```python
from build123d import *

# Parameters (mm, degrees)
SKETCH1_W           = 3.175
SKETCH1_H           = 50.8
BOSS_EXTRUDE1_DEPTH = 38.1
SKETCH3_R           = 3.175
CUT_EXTRUDE1_DEPTH  = 38.1
FILLET1_R           = 12.7


with BuildPart() as part:
    # Sketch1 → Boss-Extrude1 (new body)
    with BuildSketch(Plane.XY):
        with Locations((17.4625, -24.384)):
            Rectangle(SKETCH1_W, SKETCH1_H)
    extrude(amount=BOSS_EXTRUDE1_DEPTH)

    # Sketch3 → Cut-Extrude1 (cut)
    with BuildSketch(Plane.ZY.offset(-15.875)):
        with Locations((19.05, -24.384)):
            Circle(SKETCH3_R)
    extrude(amount=-CUT_EXTRUDE1_DEPTH, mode=Mode.SUBTRACT)

    # Fillet1
    fillet1_edges = [part.edges().sort_by_distance(p)[0] for p in [
        (17.4625, -49.784, 38.1),
        (17.4625, 1.016, 38.1),
    ]]
    fillet(fillet1_edges, radius=FILLET1_R)


solid = part.part
```
Source: CAD feature listing. Evaluate the final solid. Frame: model axes, mm. Round coordinates to 2 decimals unless told otherwise and drop trailing zeros. Write each loop counter-clockwise with the first axis right and the second up, starting at its lowest first coordinate (ties: lowest second). Pieces come first, ordered by that corner, then holes. Notation, with made-up numbers: M 50,-12.75 L 100,-12.75 A29 ccw 100,10.25 Z; hole C 4,-7 d4. An arc over 180 degrees is marked long. Answer as a JSON object with one key per item and string values. Group by question number.
(1) First-contact query: pin 1 (10 mm diameter, centred on y = -24.384, z = 19.05, fed in from -X) (3 decimals). Flat tip, straight axial feed; report the tip coordinate or a pass-through.
(2) Ray query, line 1 (Y direction, x = 17.1, z = 19.05); line 2 (Z direction, x = 16.35, y = -26.5); line 3 (Y direction, x = 18.2, z = 31.5). Return the intervals inside material, ascending. Write a range as [from, to].
(3) Section query C-C on y = -46. Output: boundary loops of the cut face in (x, z) (3 decimals), then the cut area to 3 significant figures.
(4) Section query A-A on z = 19.05. Output: boundary loops of the cut face in (x, y) (3 decimals), then the cut area to 3 significant figures.
(5) Section query B-B on x = 17.15. Output: boundary loops of the cut face in (y, z) (3 decimals).
(6) Section query D-D on z = 28.5. Output: boundary loops of the cut face in (x, y) (3 decimals).
(7) Mould query, pull axis Y, two halves, no side actions, for faces 1 (the cylindrical face through (17.44, -26.316, 16.53)), 2 (the flat face through (17, 1.016, 13)), 3 (the flat face through (17, -49.784, 13)). Classes: +Y half, -Y half, draft (parallel to the pull), parting line (faces both ways), or undercut.
Computed values:
{
 "1": {"pin 1": "x = 15.875"},
 "2": {"line 1": "[-49.78, -27.56], [-21.21, 1.02]", "line 2": "[0, 16.68], [21.42, 38.1]", "line 3": "[-48.22, -0.54]"},
 "3": {"outline": "M 15.875,0 L 19.05,0 L 19.05,34.444 L 15.875,34.444 Z", "area": "109 mm^2"},
 "4": {"outline": "M 15.875,-49.784 L 19.05,-49.784 L 19.05,-27.559 L 15.875,-27.559 Z; M 15.875,-21.209 L 19.05,-21.209 L 19.05,1.016 L 15.875,1.016 Z", "area": "141 mm^2"},
 "5": {"outline": "M -49.784,0 L 1.016,0 L 1.016,25.4 A12.7 ccw -11.684,38.1 L -37.084,38.1 A12.7 ccw -49.784,25.4 Z; hole C -24.384,19.05 d6.35"},
 "6": {"outline": "M 15.875,-49.4 L 19.05,-49.4 L 19.05,0.632 L 15.875,0.632 Z"},
 "7": {"face 1": "undercut", "face 2": "+Y half", "face 3": "-Y half"}
}
